Geometry: final body of the model. Coordinates: model frame, mm. A direction names the side the tool comes from. Give positions to 0.01 mm unless a question says otherwise; leave off trailing zeros. Loops run counter-clockwise (first coordinate to the right, second up) from the corner with the lowest first, then second, coordinate; pieces in that order, holes last.
1. Material intervals for line 1 along Y through (x, z) = (0, 6.25); line 2 along Y through (x, z) = (1, 2); line 3 along X through (y, z) = (7.25, 1.75), sorted ascending.
2. Section A-A, the plane x = 0. Output: boundary loops of the cut face in (y, z).
3. First-contact query: P1, Ø3.5, axis at y = 10.5, z = 5.5, coming from the +X side; P2, Ø10, axis at x = 1.5, y = 21, coming from the -Z side; P3, Ø2.5, axis at x = 19, z = 4, coming from the +Y side. Flat tips, straight axial feed; report the tip coordinate or a pass-through.
4. Section D-D, the plane y = 5. Output: boundary loops of the cut face in (x, z).
5. Section C-C, the plane y = 14.75. Output: boundary loops of the cut face in (x, z), then the cut area to 3 significant figures.
6. Access query for faces 1 (the face through (-20.767, 1, 4)), 2 (the face through (-17, 2.919, 4)), 3 (the face through (17, 2.919, 4)). Directions: +Z, -Z, +X, -X, +Y, -Y. A direction counts if a zero-diameter tool reaches every point of the face in a straight line with its end or side. Return the directions, or none.
7. Section B-B, the plane z = 5.5. Output: boundary loops of the cut face in (x, y), then the cut area to 3 significant figures.
8. Draft query along Y for faces 4 (the face through (10.343, 4.121, 3.944)), 5 (the face through (-0.521, 18.216, 3.944)), 6 (the face through (0, 9, 0)). Return one class per face: +Y half, -Y half, draft (parallel to the pull), parting line (faces both ways), or undercut.
from build123d import *

# Parameters (mm, degrees)
SKETCH1_R           = 4
BOSS_EXTRUDE1_DEPTH = 8


with BuildPart() as part:
    # Sketch1 → Boss-Extrude1 (new body)
    with BuildSketch(Plane.XY):
        with BuildLine():
            Line((-20.767338367, 0), (-20.767338367, 2.918605514))
            Line((-20.767338367, 2.918605514), (-13.202627173, 2.918605514))
            ThreePointArc((-13.202627173, 2.918605514), (-10.374200048, 4.090178389), (-9.202627173, 6.918605514))
            Line((-9.202627173, 6.918605514), (-9.202627173, 14.25))
            ThreePointArc((-9.202627173, 14.25), (0, 23.452627173), (9.202627173, 14.25))
            Line((9.202627173, 14.25), (9.202627173, 6.918605514))
            ThreePointArc((9.202627173, 6.918605514), (10.374200048, 4.090178389), (13.202627173, 2.918605514))
            Line((13.202627173, 2.918605514), (21.055610972, 2.918605514))
            Line((21.055610972, 2.918605514), (21.055610972, 0))
            Line((21.055610972, 0), (-20.767338367, 0))
        make_face()
        with Locations((0, 14.25)):
            Circle(SKETCH1_R, mode=Mode.SUBTRACT)
    extrude(amount=BOSS_EXTRUDE1_DEPTH)


solid = part.part
Answers below:
1. line 1: y = 0 to 10.25, 18.25 to 23.45
1. line 2: y = 0 to 10.38, 18.12 to 23.4
1. line 3: x = -9.2 to 9.2
2. outline: (0, 0) - (10.25, 0) - (10.25, 8) - (0, 8) - close; (18.25, 0) - (23.45, 0) - (23.45, 8) - (18.25, 8) - close
3. P1: stops at x = 9.2
3. P2: stops at z = 0
3. P3: stops at y = 2.92
4. outline: (-9.69, 0) - (9.69, 0) - (9.69, 8) - (-9.69, 8) - close
5. outline: (-9.19, 0) - (-3.97, 0) - (-3.97, 8) - (-9.19, 8) - close; (3.97, 0) - (9.19, 0) - (9.19, 8) - (3.97, 8) - close
5. area: 83.5 mm2
6. face 1: +Z, -Z, -X, +Y, -Y
6. face 2: +Z, -Z, -X, +Y
6. face 3: +Z, -Z, +X, +Y
7. outline: (-20.77, 0) - (21.06, 0) - (21.06, 2.92) - (13.2, 2.92) arc R4 cw to (9.2, 6.92) - (9.2, 14.25) arc R9.2 ccw to (-9.2, 14.25) - (-9.2, 6.92) arc R4 cw to (-13.2, 2.92) - (-20.77, 2.92) - close; hole circle Ø8 at (0, 14.25)
7. area: 420 mm2
8. face 4: +Y half
8. face 5: undercut
8. face 6: draft
